For this review, take the finished solid that the model builds, in its own axes (mm). Face numbers are marked on the shaded views. A direction names the side the tool comes from. Round coordinates to 2 decimals unless told otherwise and drop trailing zeros. Order: outer loops, then holes, each group sorted by start corner. A loop starts at its lowest first (then second) coordinate and runs counter-clockwise, first axis right, second up. Notation, with made-up numbers: (51.25, 84) -> (100.25, 84) arc R8 cw to (100.25, 89) -> close; hole circle Ø9 at (65, 20.5). An arc over 180 degrees is marked (long way). Use a Markdown table: item, result. Add a question column.
1) Clearance check with flat-ended pins moving along their axes: P1, Ø4, axis at x = 44.45, y = 9.98, coming from the +Z side; P2, Ø5, axis at y = 18, z = 1, coming from the +X side; P3, Ø2, axis at y = 60, z = 0, coming from the +X side; P4, Ø3, axis at y = 18, z = 1, coming from the -X side. State where each tip first meets the part, or that it passes through.
2) Consider section B-B (z = -2.75). Give the number of separate pieces and of enclosed holes in the cut face, plus the area to 3 significant figures.
3) Consider section C-C (x = 12.5). State the section outline as (y, z) points, plus the area to 3 significant figures.
4) Consider section A-A (x = 25.4). State the section outline as (y, z) points.
5) Wall thickness on line 1 along Z through (x, y) = (9.5, 13); line 2 along Y through (x, z) = (25.4, 3.15); line 3 along X through (y, z) = (7.5, 3.25): over which ranges is each line inside the solid? List them lowest first. Write a range as [from, to].
6) Consider section D-D (x = 44.45). State the section outline as (y, z) points, plus the area to 3 significant figures.
7) Machinability: for the marked faces 1 and 2, which of the approach directions +Z, -Z, +X, -X, +Y, -Y give a long, thin tool a straight path to every point of the face, cutting with its end or side? Answer none if there is none.
8) Draft analysis for pull direction Y (two halves, no side actions). For the marked faces 3, 4 and 5, state which applies: pulls with the +Y half, pulls with the -Y half, needs draft (parallel to the pull), parting line crosses it, or undercut.
```python
from build123d import *

# Parameters (mm, degrees)
SKETCH7_W           = 50.8
SKETCH7_H           = 19.05
SKETCH7_R           = 1.5875
BOSS_EXTRUDE1_DEPTH = 4.7625
SKETCH7_6_W         = 50.8
SKETCH7_6_H         = 19.05
CUT_EXTRUDE1_DEPTH  = 1.5875
SKETCH13_W          = 50.8
SKETCH13_H          = 6.35
BOSS_EXTRUDE4_DEPTH = 9.525
BOSS_EXTRUDE5_DEPTH = 9.525


with BuildPart() as part:
    # Sketch7 → Boss-Extrude1 (new, symmetric)
    with BuildSketch(Plane.XY):
        with Locations((25.4, 9.525)):
            Rectangle(SKETCH7_W, SKETCH7_H)
        with Locations(Location((25.4, 9.975665903, 0), (0, 0, 180))):
            Circle(SKETCH7_R, mode=Mode.SUBTRACT)
        with Locations(Location((44.45, 9.975665903, 0), (0, 0, 180))):
            Circle(SKETCH7_R, mode=Mode.SUBTRACT)
    extrude(amount=BOSS_EXTRUDE1_DEPTH, both=True)

    # Sketch7_6 → Cut-Extrude1 (cut, symmetric)
    with BuildSketch(Plane.XY):
        with Locations((25.4, 9.525)):
            Rectangle(SKETCH7_6_W, SKETCH7_6_H)
    extrude(amount=CUT_EXTRUDE1_DEPTH, both=True, mode=Mode.SUBTRACT)


with BuildPart() as cut_extrude1_piece_1:
    # of the separate pieces the step leaves, piece 1, a body of its own (cut_extrude1_pieces)
    add(part.part.solids().sort_by_distance((0, 0, -1.5875))[0])



with BuildPart() as cut_extrude1_piece_2:
    # of the separate pieces the step leaves, piece 2, a body of its own (cut_extrude1_pieces)
    add(part.part.solids().sort_by_distance((0, 0, 4.7625))[0])


with BuildPart() as cut_extrude1_piece_1_1:
    add(cut_extrude1_piece_1.part)

    add(cut_extrude1_piece_2.part)  # Boss-Extrude4 merges Cut-Extrude1 piece 2
    # Sketch13 → Boss-Extrude4 (add)
    with BuildSketch(Plane.XY.offset(4.7625)):
        with Locations((25.4, 22.225)):
            Rectangle(SKETCH13_W, SKETCH13_H)
    extrude(amount=-BOSS_EXTRUDE4_DEPTH)

    # Sketch14 → Boss-Extrude5 (add)
    with BuildSketch(Plane.XY.offset(4.7625)):
        with BuildLine():
            Line((50.8, 25.4), (71.902482506, 43.622575132))
            Line((71.902482506, 43.622575132), (52.787315523, 52.655864431))
            ThreePointArc((52.787315523, 52.655864431), (55.247905821, 39.572849469), (46.356867644, 29.664811055))
            ThreePointArc((46.356867644, 29.664811055), (13.014341519, 29.769386724), (-6.078550984, 57.104280913))
            ThreePointArc((-6.078550984, 57.104280913), (-4.350402215, 67.954625431), (4.26443102, 74.773798595))
            Line((4.26443102, 74.773798595), (-10.669308695, 76.446075822))
            Line((-10.669308695, 76.446075822), (-12.926576502, 54.593807627))
            Line((-12.926576502, 54.593807627), (0, 25.4))
            Line((0, 25.4), (50.8, 25.4))
        make_face()
    extrude(amount=-BOSS_EXTRUDE5_DEPTH)


solid = cut_extrude1_piece_1_1.part
```
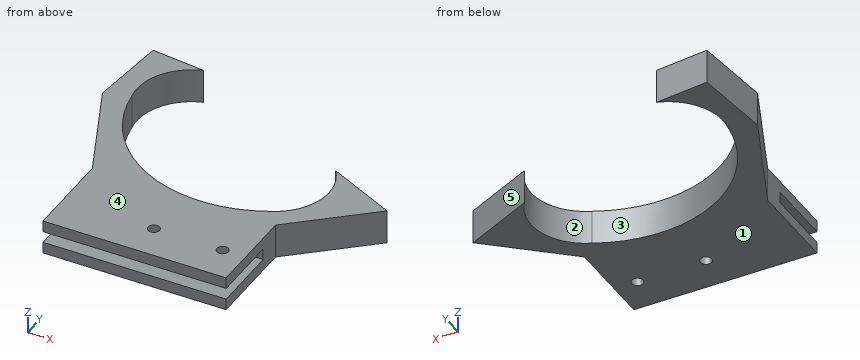
Results list:
| question | item | result |
|---|---|---|
| 1 | P1 | z = 4.76 |
| 1 | P2 | x = 50.8 |
| 1 | P3 | x = -6.37 |
| 1 | P4 | x = 0 |
| 2 | separate pieces | 1 |
| 2 | enclosed holes | 2 |
| 2 | area | 2,000 mm2 |
| 3 | outline | (0, -4.76) -> (30.04, -4.76) -> (30.04, 4.76) -> (0, 4.76) -> (0, 1.59) -> (19.05, 1.59) -> (19.05, -1.59) -> (0, -1.59) -> close |
| 3 | area | 226 mm2 |
| 4 | outline | (0, -4.76) -> (8.39, -4.76) -> (8.39, -1.59) -> (0, -1.59) -> close; (0, 1.59) -> (8.39, 1.59) -> (8.39, 4.76) -> (0, 4.76) -> close; (11.56, -4.76) -> (25.91, -4.76) -> (25.91, 4.76) -> (11.56, 4.76) -> (11.56, 1.59) -> (19.05, 1.59) -> (19.05, -1.59) -> (11.56, -1.59) -> close |
| 5 | line 1 | [-4.76, -1.59], [1.59, 4.76] |
| 5 | line 2 | [0, 8.39], [11.56, 25.91] |
| 5 | line 3 | [0, 50.8] |
| 6 | outline | (0, -4.76) -> (8.39, -4.76) -> (8.39, -1.59) -> (0, -1.59) -> close; (0, 1.59) -> (8.39, 1.59) -> (8.39, 4.76) -> (0, 4.76) -> close; (11.56, -4.76) -> (28.75, -4.76) -> (28.75, 4.76) -> (11.56, 4.76) -> (11.56, 1.59) -> (19.05, 1.59) -> (19.05, -1.59) -> (11.56, -1.59) -> close |
| 6 | area | 193 mm2 |
| 7 | face 1 | -Z, +X, -X, +Y, -Y |
| 7 | face 2 | +Z, -Z |
| 8 | face 3 | undercut |
| 8 | face 4 | needs draft |
| 8 | face 5 | pulls with the +Y half |
